For this review, take the finished solid that the model builds, in its own axes (mm). Give positions to 0.01 mm unless a question says otherwise; leave off trailing zeros. Order: outer loops, then holes, each group sorted by start corner. A loop starts at its lowest first (then second) coordinate and runs counter-clockwise, first axis right, second up. Notation, with made-up numbers: (-38, 50.25) - (0, 50.25) arc R12 cw to (0, 61.25) - close; hole circle Ø2 at (30, -29.75). An arc over 180 degrees is marked (long way). Answer as a JSON object with one key per item and string values. Group by question number.
from build123d import *

# Parameters (mm, degrees)
CROQUIS2_R              = 1.75
SALIENTE_EXTRUIR1_DEPTH = 2


with BuildPart() as part:
    # Croquis2 → Saliente-Extruir1 (new body)
    with BuildSketch(Plane(origin=(0, 0, 0), x_dir=(0, 0, -1), z_dir=(1, 0, 0))):
        with BuildLine():
            ThreePointArc((-96.614142786, 197.855252051), (-81.453806027, 262.611499523), (-75.165534077, 328.820751393))
            ThreePointArc((-75.165534077, 328.820751393), (-80.625986242, 343.931649954), (-94.904004852, 351.300094686))
            ThreePointArc((-94.904004852, 351.300094686), (-235.692785429, 360.674969525), (-376.791015079, 359.863425139))
            ThreePointArc((-376.791015079, 359.863425139), (-391.509654572, 353.355396757), (-397.859422485, 338.567792847))
            ThreePointArc((-397.859422485, 338.567792847), (-392.587269832, 222.285598409), (-369.665474686, 108.163139426))
            ThreePointArc((-369.665474686, 108.163139426), (-359.307110382, 94.973091226), (-342.66254386, 92.916033167))
            ThreePointArc((-342.66254386, 92.916033167), (-222.709683854, 132.700513572), (-107.551722613, 184.759494235))
            ThreePointArc((-107.551722613, 184.759494235), (-100.761654757, 190.203841513), (-96.614142786, 197.855252051))
        make_face()
        with Locations((-85.886008555, 339.31297425)):
            Circle(CROQUIS2_R, mode=Mode.SUBTRACT)
        with Locations((-235.905337517, 353.678197297)):
            Circle(CROQUIS2_R, mode=Mode.SUBTRACT)
        with Locations((-386.533430085, 348.4322687)):
            Circle(CROQUIS2_R, mode=Mode.SUBTRACT)
        with Locations((-385.639096494, 223.135826186)):
            Circle(CROQUIS2_R, mode=Mode.SUBTRACT)
        with Locations((-355.865347904, 101.068521567)):
            Circle(CROQUIS2_R, mode=Mode.SUBTRACT)
        with Locations((-225.256716861, 139.220684034)):
            Circle(CROQUIS2_R, mode=Mode.SUBTRACT)
        with Locations((-106.134267637, 194.691048979)):
            Circle(CROQUIS2_R, mode=Mode.SUBTRACT)
    extrude(amount=SALIENTE_EXTRUIR1_DEPTH)


solid = part.part
1) For pin 1 (12 mm diameter, centred on y = 301, z = 109.5, fed in from -X), flat-tipped, find the tip position at first contact; note if it passes through.
2) Consider section C-C (y = 217). Give the boundary of the cut face in (x, z), plus the area to 3 significant figures.
3) Consider section B-B (z = 195.5). Give the boundary of the cut face in (x, y), plus the area to 3 significant figures.
4) Consider section A-A (x = 0.65). Give the boundary of the cut face in (y, z).
5) For line 1 (Z direction, x = 0.2, y = 234.5); line 2 (Y direction, x = 1.4, z = 255.5); line 3 (Y direction, x = 1.45, z = 188), list the stretches that pass through material, from the lowest coordinate up.
Result set:
{
 "1": {"pin 1": "stops at x = 0"},
 "2": {"outline": "(0, 91.16) - (2, 91.16) - (2, 391.92) - (0, 391.92) - close", "area": "602 mm2"},
 "3": {"outline": "(0, 143.71) - (2, 143.71) - (2, 359.04) - (0, 359.04) - close", "area": "431 mm2"},
 "4": {"outline": "(92.92, 342.66) arc R1212 ccw to (184.76, 107.55) arc R22 ccw to (197.86, 96.61) arc R492 ccw to (328.82, 75.17) arc R22 ccw to (351.3, 94.9) arc R1953.6 ccw to (359.86, 376.79) arc R22 ccw to (338.57, 397.86) arc R762 ccw to (108.16, 369.67) arc R22 ccw to start; hole circle Ø3.5 at (101.07, 355.87); hole circle Ø3.5 at (139.22, 225.26); hole circle Ø3.5 at (194.69, 106.13); hole circle Ø3.5 at (223.14, 385.64); hole circle Ø3.5 at (339.31, 85.89); hole circle Ø3.5 at (348.43, 386.53); hole circle Ø3.5 at (353.68, 235.91)"},
 "5": {"line 1": "z = 86.9 to 393.98", "line 2": "y = 120.43 to 361.18", "line 3": "y = 146.88 to 358.64"}
}
